Autodesk Inventor part; units mm, degrees
ref_plane "YZ Plane" through (0, 0, 0) normal (1, 0, 0) x (0, 1, 0)
ref_plane "XZ Plane" through (0, 0, 0) normal (0, 1, 0) x (-1, 0, 0)
ref_plane "XY Plane" through (0, 0, 0) normal (0, 0, 1) x (1, 0, 0)
sketch "Skizze1" plane through (0, 0, 0) normal (0, 1, 0) x (-1, 0, 0)
  line L0 (0, 0) -> (15, 0)
  line L1 (15, 0) -> (15, -40)
  line L2 (15, -40) -> (0, -40)
  line L3 (0, -40) -> (0, 0)
  dimension "d0" = 15
  dimension "d1" = 40
extrude "Extrusion1" add sketch "Skizze1" along normal blind 5
fillet "Rundung1" radius 1 4 edges at (-15, 2.5, 0) (0, 2.5, 0) (0, 2.5, -40) (-15, 2.5, -40)
sketch "Skizze2" plane through (0, 0, 0) normal (0, -1, 0) x (1, 0, 0)
  line L0 (-1, 0) -> (-14, 0)
  line L1 (0, -39) -> (0, -1)
  line L2 (-14, -40) -> (-1, -40)
  point P0 (0, 0)
  point P1 (-7.5, -5)
  point P2 (-7.5, -35)
  dimension "d5" = 5
  dimension "d6" = 5
  dimension "d7" = 7.5
  dimension "d8" = 7.5
  dimension "d9" = 30
hole "Bohrung1" at (-7.5, 0, -5) at (-7.5, 0, -35) direction (0, 1, 0) diameter 4 end through all
sketch "Skizze3" plane through (0, 0, 0) normal (0, -1, 0) x (1, 0, 0)
  line L0 (-1, 0) -> (-14, 0)
  line L1 (0, -39) -> (0, -1)
  point P0 (0, 0)
  point P1 (-7.5, -20)
  dimension "d17" = 20
  dimension "d18" = 7.5
properties part number "halter_test"
Input: part model. Units: mm. Frame: model coordinates. Coordinates: 2 decimals unless noted, no trailing zeros. Loops run counter-clockwise (first coordinate to the right, second up) from the corner with the lowest first, then second, coordinate; pieces in that order, holes last.
Q1. Line query: line 1 along X through (y, z) = (1.75, -35); line 2 along Z through (x, y) = (-7.5, 1); line 3 along Z through (x, y) = (-8.5, 3). Output: solid intervals per line, ascending.
Results are:
line 1: x = -15 to -9.5, -5.5 to 0
line 2: z = -40 to -37, -33 to -7, -3 to 0
line 3: z = -40 to -36.73, -33.27 to -6.73, -3.27 to 0
Q2. Mould query, pull axis Z, two halves, no side actions, for faces 1 (the cylindrical face through (-8.852, 2.535, -3.526)), 2 (the flat face through (-15, 2, -20)), 3 (the flat face through (-7, 2, 0)), 4 (the flat face through (-8, 2, -40)). Classes: +Z half, -Z half, draft (parallel to the pull), parting line (faces both ways), or undercut.
Results are:
face 1: undercut
face 2: draft
face 3: +Z half
face 4: -Z half
Q3. Section C-C, the plane y = 2.7. Return the cut outline in (x, z), and give its area (3 significant figures).
Results are:
outline: (-15, -39) arc R1 ccw to (-14, -40) - (-1, -40) arc R1 ccw to (0, -39) - (0, -1) arc R1 ccw to (-1, 0) - (-14, 0) arc R1 ccw to (-15, -1) - close; hole circle Ø4 at (-7.5, -35); hole circle Ø4 at (-7.5, -5)
area: 574 mm2
Q4. Section B-B, the plane x = -7.5. Return the cut outline in (y, z).
Results are:
outline: (0, -40) - (5, -40) - (5, -37) - (0, -37) - close; (0, -33) - (5, -33) - (5, -7) - (0, -7) - close; (0, -3) - (5, -3) - (5, 0) - (0, 0) - close
Q5. Section A-A, the plane z = -35. Return the cut outline in (x, y).
Results are:
outline: (-15, 0) - (-9.5, 0) - (-9.5, 5) - (-15, 5) - close; (-5.5, 0) - (0, 0) - (0, 5) - (-5.5, 5) - close
Q6. Contact query for a flat-ended pin moving along its axis: pin 1 (6.5 mm diameter, centred on x = -7.5, z = -35, fed in from -Y). Output: stop coordinate, or through.
Results are:
pin 1: stops at y = 0
